```python
from build123d import *

# Parameters (mm, degrees)
F0_W         = 30.48
F0_H         = 30.48
F0_W_2       = 25.4
F0_H_2       = 25.4
F1_DEPTH     = 3.81
F0_W_3       = 15.24
F0_H_3       = 15.24
F2_DEPTH     = 20.32
F3_DEPTH     = 2.54
F4_T4_DEPTH  = 131.0338200082
F4_T9_DEPTH  = 131.0338200082
F4_T14_DEPTH = 131.0338200082
F4_T19_DEPTH = 131.0338200082


# Not quite as in the source:
# - a fillet or chamfer that OpenCascade refuses, or shapes differently, is made with other operations: its cross-section is extruded or revolved along the edge and cut away or added


with BuildPart() as f1:
    # F0 (on Front) → F1 (new body)
    with BuildSketch(Plane.XZ):
        Rectangle(F0_W, F0_H)
        Rectangle(F0_W_2, F0_H_2, mode=Mode.SUBTRACT)
    extrude(amount=F1_DEPTH)

    # F0 (on Front) → F2 (join)
    with BuildSketch(Plane.XZ):
        Rectangle(F0_W_2, F0_H_2)
        Rectangle(F0_W_3, F0_H_3, mode=Mode.SUBTRACT)
        Rectangle(F0_W_3, F0_H_3)
    extrude(amount=F2_DEPTH)

    # F0 (on Front) → F3 (cut)
    with BuildSketch(Plane.XZ):
        Rectangle(F0_W_2, F0_H_2)
        Rectangle(F0_W_3, F0_H_3, mode=Mode.SUBTRACT)
        Rectangle(F0_W_3, F0_H_3)
    extrude(amount=F3_DEPTH, mode=Mode.SUBTRACT)

    # F4: chamfer of 2.54 x 20.32 on 4 edges, made by hand


with BuildPart() as f4_tool2:
    # F4_s3 → F4_t4 (new body)
    with BuildSketch(Plane.YZ.offset(65.5169100041)):
        Polygon((0, 12.7), (-20.32, 10.16), (-20.32, 12.7), align=None)
    extrude(amount=-F4_T4_DEPTH)

    split(bisect_by=Plane.XZ.offset(3.81), keep=Keep.TOP)


with BuildPart() as f1_1:
    add(f1.part)

    # F4_t1: cut F4_tool2
    add(f4_tool2.part, mode=Mode.SUBTRACT)


with BuildPart() as f4_tool7:
    # F4_s8 → F4_t9 (new body)
    with BuildSketch(Plane.XY.offset(65.5169100041)):
        Polygon((-12.7, 0), (-10.16, -20.32), (-12.7, -20.32), align=None)
    extrude(amount=-F4_T9_DEPTH)

    split(bisect_by=Plane.XZ.offset(3.81), keep=Keep.TOP)


with BuildPart() as f1_2:
    add(f1_1.part)

    # F4_t6: cut F4_tool7
    add(f4_tool7.part, mode=Mode.SUBTRACT)


with BuildPart() as f4_tool12:
    # F4_s13 → F4_t14 (new body)
    with BuildSketch(Plane.YZ.offset(-65.5169100041)):
        Polygon((0, -12.7), (-20.32, -10.16), (-20.32, -12.7), align=None)
    extrude(amount=F4_T14_DEPTH)

    split(bisect_by=Plane.XZ.offset(3.81), keep=Keep.TOP)


with BuildPart() as f1_3:
    add(f1_2.part)

    # F4_t11: cut F4_tool12
    add(f4_tool12.part, mode=Mode.SUBTRACT)


with BuildPart() as f4_tool17:
    # F4_s18 → F4_t19 (new body)
    with BuildSketch(Plane.XY.offset(-65.5169100041)):
        Polygon((12.7, 0), (10.16, -20.32), (12.7, -20.32), align=None)
    extrude(amount=F4_T19_DEPTH)

    split(bisect_by=Plane.XZ.offset(3.81), keep=Keep.TOP)


with BuildPart() as f1_4:
    add(f1_3.part)

    # F4_t16: cut F4_tool17
    add(f4_tool17.part, mode=Mode.SUBTRACT)


solid = f1_4.part
```
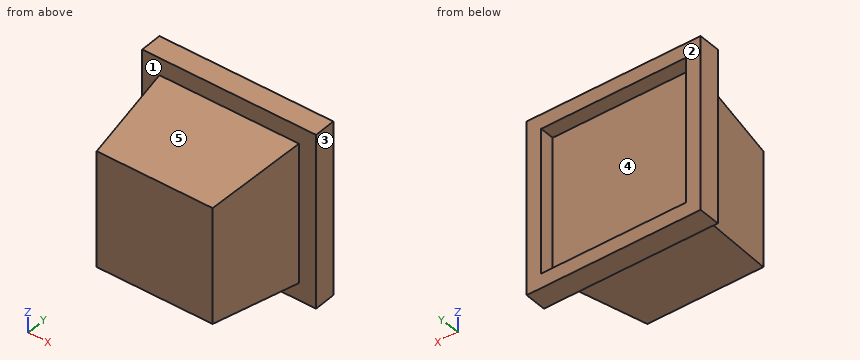
Here's how the part is built. I have some questions about the finished solid (model axes, mm). Face numbers are marked on the shaded views. A direction names the side the tool comes from. Round coordinates to 2 decimals unless told otherwise and drop trailing zeros. Write each loop counter-clockwise with the first axis right and the second up, starting at its lowest first coordinate (ties: lowest second). Pieces come first, ordered by that corner, then holes. Notation, with made-up numbers: M -9,49 L 8,49 A18 cw 8,82 Z; hole C 41,22.25 d2. An arc over 180 degrees is marked long. Answer as CSV lines item,"result". Start each with the question number.
1. Suppose I cut it at C-C on y = -1.5. Write out the boundary of the cut face in (x, z), then the cut area to 3 significant figures.
2. I'm going to push flat-ended pins straight in: pin 1 Ø8 at (x, y) = (5.5, -17) entering from -Z (3 decimals); pin 2 Ø1.5 at (y, z) = (-14, -10.5) entering from +X; pin 3 Ø4 at (y, z) = (-9, -7.5) entering from +X (3 decimals). Where does each tip first touch, or does it pass through?
3. Suppose I cut it at A-A on x = 3. Write out the boundary of the cut face in (y, z), then the cut area to 3 significant figures.
4. Thinking about a two-plate mould opening in X: for the marked faces 3, 4 and 5, which applies, released by +X, released by -X, zero draft, split by the parting line, or undercut?
5. Suppose I cut it at B-B on z = 7. Write out the boundary of the cut face in (x, y), then the cut area to 3 significant figures.
6. Suppose I cut it at D-D on y = -9. Write out the boundary of the cut face in (x, z) (3 decimals), then the cut area to 3 significant figures.
7. I need wall thicknesses on probe 1 along Z at (x, y) = (6, -2); probe 2 along Y at (x, z) = (-6.5, -6.5); probe 3 along Y at (x, z) = (13, -6.5). Which ranges of each line are inside material? Lowest first, please.
8. On a 3-axis mill with a long thin cutter (end or side, diameter ignored), from which of +Z, -Z, +X, -X, +Y, -Y can I reach the whole of each face in a straight line? I mean the marked faces 1 and 2. Say none if no direction works.
Check result:
1,outline,"M -15.24,-15.24 L 15.24,-15.24 L 15.24,15.24 L -15.24,15.24 Z; hole M -12.7,-12.7 L 12.7,-12.7 L 12.7,12.7 L -12.7,12.7 Z"
1,area,"284 mm2"
2,pin 1,"stops at z = -11.075"
2,pin 2,"stops at x = 11.04"
2,pin 3,"stops at x = 11.825"
3,outline,"M -20.32,-10.16 L -3.81,-12.22 L -3.81,-15.24 L 0,-15.24 L 0,-12.7 L -2.54,-12.7 L -2.54,12.7 L 0,12.7 L 0,15.24 L -3.81,15.24 L -3.81,12.22 L -20.32,10.16 Z"
3,area,"421 mm2"
4,face 3,"released by +X"
4,face 4,"undercut"
4,face 5,"zero draft"
5,outline,"M -15.24,-3.81 L -12.22,-3.81 L -10.16,-20.32 L 10.16,-20.32 L 12.22,-3.81 L 15.24,-3.81 L 15.24,0 L 12.7,0 L 12.7,-2.54 L -12.7,-2.54 L -12.7,0 L -15.24,0 Z"
5,area,"421 mm2"
6,outline,"M -11.575,-11.575 L 11.575,-11.575 L 11.575,11.575 L -11.575,11.575 Z"
6,area,"536 mm2"
7,probe 1,"z = -15.24 to -12.7, 12.7 to 15.24"
7,probe 2,"y = -20.32 to -2.54"
7,probe 3,"y = -3.81 to 0"
8,face 1,"-Y"
8,face 2,"+Z, -Z, +X, -X, +Y"
